from build123d import *

# Parameters (mm, degrees)
DIAPROFILES_R         = 6
DIAPROFILES_R_2       = 5.5
DIAPROFILE_DEPTH      = 1.5
BEARINGPATHPROFILES_R = 0.7


with BuildPart() as part:
    # DiaProfileS → DiaProfile (new, symmetric)
    with BuildSketch(Plane(origin=(0, 0, 0), x_dir=(1, 0, 0), z_dir=(0, 1, 0))):
        with Locations(Location((0, 0, 0), (0, 0, 270))):
            Circle(DIAPROFILES_R)
        with Locations(Location((0, 0, 0), (0, 0, 270))):
            Circle(DIAPROFILES_R_2, mode=Mode.SUBTRACT)
    extrude(amount=DIAPROFILE_DEPTH, both=True)

    # BearingPathProfileS → BearingPathProfile (revolve, cut)
    with BuildSketch(Plane.XY, mode=Mode.PRIVATE) as bearingpathprofile_sk:
        with Locations((5, 0)):
            Circle(BEARINGPATHPROFILES_R)
    revolve(bearingpathprofile_sk.sketch.rotate(Axis((0, 1.5, 0), (0, -1, 0)), 90), axis=Axis((0, 1.5, 0), (0, -1, 0)), mode=Mode.SUBTRACT)


solid = part.part
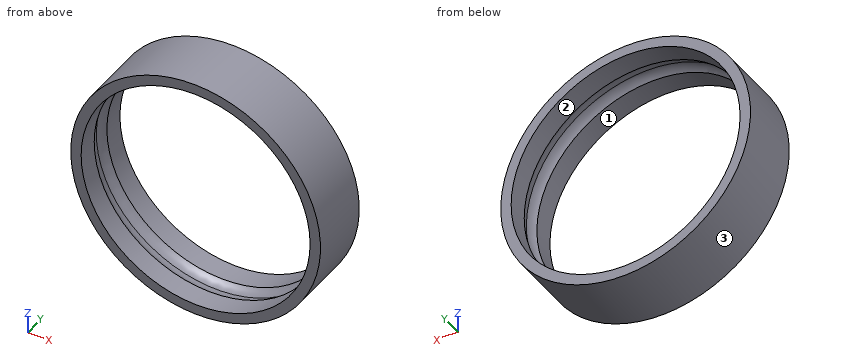
Could you check a few things on this model? Use its own coordinates, in mm. Face numbers are marked on the shaded views. Round coordinates to 2 decimals unless told otherwise and drop trailing zeros. Order: outer loops, then holes, each group sorted by start corner. A loop starts at its lowest first (then second) coordinate and runs counter-clockwise, first axis right, second up. Notation, with made-up numbers: M 9,16 L 42,16 A9 cw 42,28 Z; hole C 67,10.5 d8. An arc over 180 degrees is marked long. One line per item, written item: value.
(1) Imagine slicing it at B-B (z = 0). Write out the boundary of the cut face in (x, y).
Ans:
outline: M -6,-1.5 L -5.5,-1.5 L -5.5,-0.49 A0.7 cw -5.5,0.49 L -5.5,1.5 L -6,1.5 Z; M 5.5,-1.5 L 6,-1.5 L 6,1.5 L 5.5,1.5 L 5.5,0.49 A0.7 cw 5.5,-0.49 Z
(2) Imagine slicing it at A-A (x = 0). Write out the boundary of the cut face in (y, z).
Ans:
outline: M -1.5,-6 L 1.5,-6 L 1.5,-5.5 L 0.49,-5.5 A0.7 cw -0.49,-5.5 L -1.5,-5.5 Z; M -1.5,5.5 L -0.49,5.5 A0.7 cw 0.49,5.5 L 1.5,5.5 L 1.5,6 L -1.5,6 Z
(3) If we mould it in two halves opening along X, with no side actions, what happens to the marked faces 1, 2 and 3? For each: released by +X, released by -X, zero draft, split by the parting line, or undercut.
Ans:
face 1: undercut
face 2: undercut
face 3: split by the parting line
(4) I'm going to push flat-ended pins straight in: P1, Ø1.5, axis at y = 0.5, z = -2, coming from the -X side; P2, Ø1.5, axis at x = 4, y = -0.5, coming from the -Z side; P3, Ø1, axis at y = -1, z = 2.5, coming from the +X side. Where does each tip first touch, or does it pass through?
Ans:
P1: stops at x = -5.87
P2: stops at z = -5.04
P3: stops at x = 5.66
(5) I need wall thicknesses on line 1 along X through (y, z) = (-1.2, 0); line 2 along X through (y, z) = (-0.2, -4.5); line 3 along Z through (x, y) = (-0.25, 1.05). Which ranges of each line are inside material? Lowest first, please. Write a range as from..to.
Ans:
line 1: x = -6..-5.5, 5.5..6
line 2: x = -3.97..-3.45, 3.45..3.97
line 3: z = -5.99..-5.49, 5.49..5.99
(6) Imagine slicing it at C-C (y = 1.3). Write out the boundary of the cut face in (x, z), and give its area (3 significant figures).
Ans:
outline: C 0,0 d12; hole C 0,0 d11
area: 18.1 mm^2
